Verification items for the finished model (mm, model axes). Give positions to 0.01 mm unless a question says otherwise; leave off trailing zeros. Order: outer loops, then holes, each group sorted by start corner. A loop starts at its lowest first (then second) coordinate and runs counter-clockwise, first axis right, second up. Notation, with made-up numbers: (9, -29.5) -> (39, -29.5) arc R24 cw to (39, -18.5) -> close; hole circle Ø1 at (30, -32). An arc over 180 degrees is marked (long way). Return JSON: item names as keys, results as strings. Group by question number.
(1) Cross-section at B-B on z = -2.25. Enter the section's corners in (x, y) (1 decimal), then the cut area to 3 significant figures.
(2) Cross-section at A-A on y = 0. Enter the section's corners in (x, z).
(3) Thickness scan on line 1 along X through (y, z) = (2.75, -0.5); line 2 along X through (y, z) = (1.25, -1.75). Record the ranges inside material, lowest first.
(4) Release check for a two-part mould opening along Y. For faces 1 (the face through (-1, 0, -6.35)), 2 (the face through (-43.66, 0.17, -3.22)), 3 (the face through (-1, 12.7, -3)) record: pulls with the +Y half, pulls with the -Y half, needs draft (parallel to the pull), parting line crosses it, or undercut.
from build123d import *

# Parameters (mm, degrees)
F0_W     = 127
F0_H     = 25.4
F1_DEPTH = 6.35
F2_R     = 1.27
F4_D     = 7.9375


with BuildPart() as f1:
    # F0 (on Top) → F1 (new body)
    with BuildSketch(Plane.XY):
        Rectangle(F0_W, F0_H)
    extrude(amount=-F1_DEPTH)

    # F2
    f2_edges = [f1.edges().sort_by_distance(p)[0] for p in [
        (-63.5, -12.7, -3.175),
        (-63.5, 12.7, -3.175),
        (63.5, 12.7, -3.175),
        (63.5, -12.7, -3.175),
    ]]
    fillet(f2_edges, radius=F2_R)

    # F4 (through all)
    with Locations(Plane.XY):
        with Locations((-47.625, 0), (47.625, 0)):
            Hole(F4_D / 2)


solid = f1.part
Verdict:
{
 "1": {"outline": "(-63.5, -11.4) arc R1.3 ccw to (-62.2, -12.7) -> (62.2, -12.7) arc R1.3 ccw to (63.5, -11.4) -> (63.5, 11.4) arc R1.3 ccw to (62.2, 12.7) -> (-62.2, 12.7) arc R1.3 ccw to (-63.5, 11.4) -> close; hole circle Ø7.9 at (-47.6, 0); hole circle Ø7.9 at (47.6, 0)", "area": "3,130 mm²"},
 "2": {"outline": "(-63.5, -6.35) -> (-51.59, -6.35) -> (-51.59, 0) -> (-63.5, 0) -> close; (-43.66, -6.35) -> (43.66, -6.35) -> (43.66, 0) -> (-43.66, 0) -> close; (51.59, -6.35) -> (63.5, -6.35) -> (63.5, 0) -> (51.59, 0) -> close"},
 "3": {"line 1": "-63.5 to -50.49, -44.76 to 44.76, 50.49 to 63.5", "line 2": "-63.5 to -51.39, -43.86 to 43.86, 51.39 to 63.5"},
 "4": {"face 1": "needs draft", "face 2": "undercut", "face 3": "pulls with the +Y half"}
}
